```python
from build123d import *

# Parameters (mm, degrees)
SKETCH1_W                = 279.4
SKETCH1_H                = 38.1
BOSS_EXTRUDE1_DEPTH      = 31.75
BOSS_EXTRUDE1_DEPTH_BACK = 31.75
SKETCH2_W                = 85.344
SKETCH2_H                = 85.344
BOSS_EXTRUDE2_DEPTH      = 38.1
CUT_EXTRUDE3_DEPTH       = 86.3440001
CUT_EXTRUDE4_DEPTH       = 140.7
CUT_EXTRUDE4_DEPTH_BACK  = 140.7
CUT_EXTRUDE5_DEPTH       = 280.4


with BuildPart() as part:
    # Sketch1 → Boss-Extrude1 (new body, two sides)
    with BuildSketch(Plane.XY) as boss_extrude1_sk:
        Rectangle(SKETCH1_W, SKETCH1_H)
    extrude(amount=BOSS_EXTRUDE1_DEPTH)
    extrude(boss_extrude1_sk.sketch, amount=-BOSS_EXTRUDE1_DEPTH_BACK)

    # Sketch2 → Boss-Extrude2 (add)
    with BuildSketch(Plane.XZ.offset(19.05)):
        Rectangle(SKETCH2_W, SKETCH2_H)
    extrude(amount=BOSS_EXTRUDE2_DEPTH)

    # Sketch3 → Cut-Revolve8 (revolve, cut)
    with BuildSketch(Plane.XY):
        with BuildLine():
            Line((-42.672, -49.517710244), (-67.10297317, -49.517710244))
            Line((-67.10297317, -49.517710244), (-67.10297317, -19.05))
            Line((-67.10297317, -19.05), (-6.167552681, -19.05))
            add(Edge.make_bspline(
                [(-42.672, -49.517710244), (-14.406584367, -46.12312834), (-6.167552681, -19.05)],
                knots=[0, 0, 0, 1, 1, 1], degree=2))
        make_face()
    revolve(axis=Axis((0, -19.05, 0), (0, -1, 0)), mode=Mode.SUBTRACT)

    # Sketch5 → Cut-Extrude3 (cut, through all)
    with BuildSketch(Plane.XY.offset(42.672)):
        Polygon((-38.1, -57.15), (-42.672, -49.517710244), (-42.672, -57.15), align=None)
        Polygon((38.1, -57.15), (42.672, -49.517710244), (42.672, -57.15), align=None)
    extrude(amount=-CUT_EXTRUDE3_DEPTH, mode=Mode.SUBTRACT)

    # Sketch6 → Cut-Extrude4 (cut, two sides)
    with BuildSketch(Plane(origin=(0, 0, 0), x_dir=(0, 0, -1), z_dir=(1, 0, 0))) as cut_extrude4_sk:
        Polygon((-42.672, -49.517710244), (-42.672, -57.15), (-38.1, -57.15), align=None)
        Polygon((42.672, -49.517710244), (42.672, -57.15), (38.1, -57.15), align=None)
    extrude(amount=CUT_EXTRUDE4_DEPTH, mode=Mode.SUBTRACT)
    extrude(cut_extrude4_sk.sketch, amount=-CUT_EXTRUDE4_DEPTH_BACK, mode=Mode.SUBTRACT)

    # Sketch7 → Cut-Extrude5 (cut, through all)
    with BuildSketch(Plane(origin=(139.7, 0, 0), x_dir=(0, 0, -1), z_dir=(1, 0, 0))):
        with BuildLine():
            Line((-29.778395533, 19.05), (-31.75, 19.05))
            Line((-31.75, 19.05), (-31.75, -19.05))
            Line((-31.75, -19.05), (-29.778395533, -19.05))
            add(Edge.make_bspline(
                [(-29.778395533, 19.05), (-33.222300303, -0.003701855), (-29.778395533, -19.05)],
                knots=[0, 0, 0, 1, 1, 1], degree=2))
        make_face()
    extrude(amount=-CUT_EXTRUDE5_DEPTH, mode=Mode.SUBTRACT)


solid = part.part
```
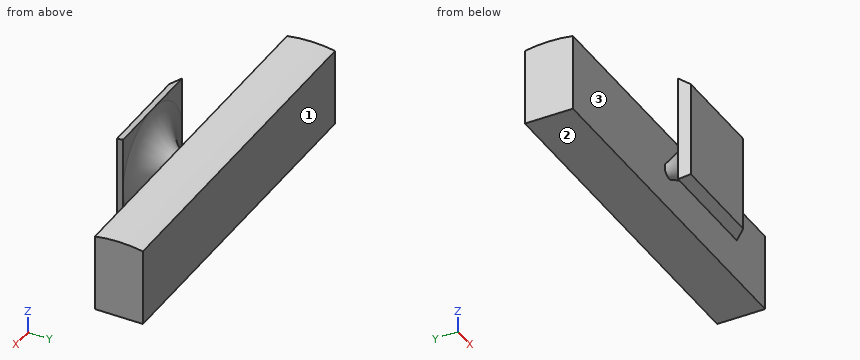
Design review of the part built by this model. Coordinates are the model's own, in mm. Face numbers are marked on the shaded views. Give positions to 0.01 mm unless a question says otherwise; leave off trailing zeros. Answer in a Markdown table with one row per item.
(1) Mouldability with a two-part tool opening along Y and no side actions: class the marked faces 1, 2 and 3 as +Y half, -Y half, draft (parallel to the pull), parting line (faces both ways), or undercut.
Results:
| item | result |
|---|---|
| face 1 | +Y half |
| face 2 | draft |
| face 3 | undercut |
(2) Clearance check with flat-ended pins moving along their axes: pin 1 (1.5 mm diameter, centred on y = -2, z = 33.5, fed in from +X); pin 2 (2 mm diameter, centred on x = -101.5, z = 20, fed in from -Y); pin 3 (1.5 mm diameter, centred on x = -76, y = -7.5, fed in from +Z); pin 4 (1.5 mm diameter, centred on x = 32, y = 10.5, fed in from -Z). State where each tip first meets the part, or that it passes through.
Results:
| item | result |
|---|---|
| pin 1 | through |
| pin 2 | y = -19.05 |
| pin 3 | z = 31.28 |
| pin 4 | z = -31.75 |
(3) To check wall thickness, follow probe 1 along Y at (x, z) = (-76, 17.5); probe 2 along Y at (x, z) = (37.5, 16.5); probe 3 along Z at (x, y) = (6.5, -30). State the ranges of each line that lie inside material, in increasing order.
Results:
| item | result |
|---|---|
| probe 1 | -19.05 to 19.05 |
| probe 2 | -57.15 to -49.29, -19.05 to 19.05 |
| probe 3 | -8.71 to 8.71 |
